Part model, mm, in its own coordinate system. A direction names the side the tool comes from. Coordinates: 2 decimals unless noted, no trailing zeros. Write each loop counter-clockwise with the first axis right and the second up, starting at its lowest first coordinate (ties: lowest second). Pieces come first, ordered by that corner, then holes. Notation, with made-up numbers: M 7,-39 L 53,-39 A24 ccw 53,-6 Z; hole C 68,-34.75 d9. An arc over 180 degrees is marked long. Use a Markdown table: item, result. Add a question column.
Q1. Mould opens along Z. For faces 4 (the flat face through (399, 30, -878)), 5 (the flat face through (100, 50, -592)) say: released by +Z, released by -Z, zero draft, split by the parting line, or undercut.
Q2. Tool access for faces 1 (the flat face through (573, 130, -599)), 2 (the flat face through (633, 145, -878)), 3 (the flat face through (394, 99, -100)): list every direction of +Z, -Z, +X, -X, +Y, -Y with a clear straight run to the whole face (end or side of a thin tool).
Q3. Wall check: L1, parallel to Z at x = 567, y = 133.5; L2, parallel to X at y = 77, z = -564.5; L3, parallel to Y at x = 440, z = -174. Give the ranges that are in metal, low to high. Write a range as from..to.
Q4. Slice it at B-B on y = 77. Count the separate pieces of the cut face and the enclosed holes in it, then the cut area to 3 significant figures.
Q5. Slice it at C-C on x = 286.5. Write the cut outline in (y, z), then the cut area to 3 significant figures.
Q6. Slice it at A-A on x = 59.5. Write the cut outline in (y, z), then the cut area to 3 significant figures.
Q7. Pin check, flat tip, straight feed: pin 1 Ø8.5 at (x, z) = (228, -1130.5) entering from +Y. Stop position of the tip, or through.
from build123d import *

# Parameters (mm, degrees)
SKETCH1_W           = 800
SKETCH1_H           = 1200
BOSS_EXTRUDE1_DEPTH = 160
SKETCH2_W           = 250
SKETCH2_H           = 130
CUT_EXTRUDE1_DEPTH  = 1452.068571777
SKETCH3_W           = 450
SKETCH3_H           = 115
CUT_EXTRUDE2_DEPTH  = 1452.068571777
SKETCH4_W           = 16.666666667
SKETCH4_H           = 15
SKETCH4_W_2         = 16.666666666
CUT_EXTRUDE3_DEPTH  = 1452.068571777


with BuildPart() as part:
    # Sketch1 → Boss-Extrude1 (new body)
    with BuildSketch(Plane(origin=(0, 0, 0), x_dir=(1, 0, 0), z_dir=(0, 1, 0))):
        with Locations((400, 600)):
            Rectangle(SKETCH1_W, SKETCH1_H)
    extrude(amount=BOSS_EXTRUDE1_DEPTH)

    # Sketch2 → Cut-Extrude1 (cut, through all)
    with BuildSketch(Plane.XY):
        with Locations((225, 65)):
            Rectangle(SKETCH2_W, SKETCH2_H)
        with Locations((575, 65)):
            Rectangle(SKETCH2_W, SKETCH2_H)
    extrude(amount=-CUT_EXTRUDE1_DEPTH, mode=Mode.SUBTRACT)

    # Sketch3 → Cut-Extrude2 (cut, through all)
    with BuildSketch(Plane.ZY):
        with Locations((-875, 87.5)):
            Rectangle(SKETCH3_W, SKETCH3_H)
        with Locations((-325, 87.5)):
            Rectangle(SKETCH3_W, SKETCH3_H)
    extrude(amount=-CUT_EXTRUDE2_DEPTH, mode=Mode.SUBTRACT)

    # Sketch4 → Cut-Extrude3 (cut, through all)
    with BuildSketch(Plane.XY):
        with Locations((108.333333334, 152.5)):
            Rectangle(SKETCH4_W, SKETCH4_H)
        with Locations((225, 152.5)):
            Rectangle(SKETCH4_W_2, SKETCH4_H)
        with Locations((341.666666667, 152.5)):
            Rectangle(SKETCH4_W, SKETCH4_H)
        with Locations((458.333333334, 152.5)):
            Rectangle(SKETCH4_W, SKETCH4_H)
        with Locations((575, 152.5)):
            Rectangle(SKETCH4_W_2, SKETCH4_H)
        with Locations((691.666666667, 152.5)):
            Rectangle(SKETCH4_W, SKETCH4_H)
    extrude(amount=-CUT_EXTRUDE3_DEPTH, mode=Mode.SUBTRACT)


solid = part.part
Recorded:
| question | item | result |
|---|---|---|
| 1 | face 4 | undercut |
| 1 | face 5 | zero draft |
| 2 | face 1 | +Z, -Z, -Y |
| 2 | face 2 | +X, -X, -Y |
| 2 | face 3 | +X, -X |
| 3 | L1 | -1200..-1100, -650..-550, -100..0 |
| 3 | L2 | 0..100, 350..450, 700..800 |
| 3 | L3 | 0..30, 145..160 |
| 4 | separate pieces | 9 |
| 4 | enclosed holes | 0 |
| 4 | area | 90,000 mm² |
| 5 | outline | M 130,-1200 L 160,-1200 L 160,0 L 130,0 L 130,-100 L 145,-100 L 145,-550 L 130,-550 L 130,-650 L 145,-650 L 145,-1100 L 130,-1100 Z |
| 5 | area | 22,500 mm² |
| 6 | outline | M 0,-1200 L 160,-1200 L 160,0 L 0,0 Z; hole M 30,-1100 L 145,-1100 L 145,-650 L 30,-650 Z; hole M 30,-550 L 145,-550 L 145,-100 L 30,-100 Z |
| 6 | area | 88,500 mm² |
| 7 | pin 1 | y = 145 |
